The listing builds one solid part. Answer for the finished solid, in the listing's coordinates (mm). A direction names the side the tool comes from. Coordinates: 2 decimals unless noted, no trailing zeros. Order: outer loops, then holes, each group sorted by start corner. A loop starts at its lowest first (then second) coordinate and runs counter-clockwise, first axis right, second up. Notation, with made-up numbers: (-16, 42.5) -> (33, 42.5) arc R13 cw to (33, 66.5) -> close; hole circle Ø9 at (-14, -30). An arc over 180 degrees is marked (long way). Write item = value, one per line.
from build123d import *

# Parameters (mm, degrees)
CYLINDER127_R             = 1.6
CYLINDER127_DEPTH         = 25
CYLINDER126_R             = 1.6
CYLINDER126_DEPTH         = 25
CYLINDER128_R             = 1.6
CYLINDER128_DEPTH         = 25
CYLINDER129_R             = 1.6
CYLINDER129_DEPTH         = 25
FUSION106_PLACEMENT_ANGLE = 3
BOX058_W                  = 8
BOX058_H                  = 8
BOX058_DEPTH              = 50
BOX057_W                  = 110
BOX057_H                  = 10
BOX057_DEPTH              = 10
BOX059_W                  = 10
BOX059_H                  = 10
BOX059_DEPTH              = 50
BOX056_W                  = 110
BOX056_H                  = 10
BOX056_DEPTH              = 10
FILLET026_R               = 9.99
FILLET026_PLACEMENT_ANGLE = 3


with BuildPart() as cylinder127:
    # Cylinder127 → Cylinder127 (new body)
    with BuildSketch(Plane(origin=(76.5, 96, 46.5), x_dir=(1, 0, 0), z_dir=(0, -1, 0))):
        Circle(CYLINDER127_R)
    extrude(amount=CYLINDER127_DEPTH)


with BuildPart() as cylinder126:
    # Cylinder126 → Cylinder126 (new body)
    with BuildSketch(Plane(origin=(76.5, 96, 3.5), x_dir=(1, 0, 0), z_dir=(0, -1, 0))):
        Circle(CYLINDER126_R)
    extrude(amount=CYLINDER126_DEPTH)


with BuildPart() as cylinder128:
    # Cylinder128 → Cylinder128 (new body)
    with BuildSketch(Plane(origin=(3.5, 96, 46.5), x_dir=(1, 0, 0), z_dir=(0, -1, 0))):
        Circle(CYLINDER128_R)
    extrude(amount=CYLINDER128_DEPTH)


with BuildPart() as fusion106:
    # Cylinder129 → Cylinder129 (new body)
    with BuildSketch(Plane(origin=(3.5, 96, 3.5), x_dir=(1, 0, 0), z_dir=(0, -1, 0))):
        Circle(CYLINDER129_R)
    extrude(amount=CYLINDER129_DEPTH)

    # Fusion106: union Cylinder127, Cylinder126, Cylinder128
    add(cylinder127.part)
    add(cylinder126.part)
    add(cylinder128.part)


with BuildPart() as fusion106_1:
    # Fusion106 placement: moved
    add(fusion106.part.moved(Location((306, -120, -55))).rotate(Axis((306, -120, -55), (0, -1, 0)), FUSION106_PLACEMENT_ANGLE))


with BuildPart() as cube037:
    # Box058 → Box058 (new body)
    with BuildSketch(Plane(origin=(100, 2, -40), x_dir=(1, 0, 0), z_dir=(0, 0, 1))):
        with Locations((4, 4)):
            Rectangle(BOX058_W, BOX058_H)
    extrude(amount=BOX058_DEPTH)


with BuildPart() as cube036:
    # Box057 → Box057 (new body)
    with BuildSketch(Plane.XY.offset(-40)):
        with Locations((55, 5)):
            Rectangle(BOX057_W, BOX057_H)
    extrude(amount=BOX057_DEPTH)


with BuildPart() as cube038:
    # Box059 → Box059 (new body)
    with BuildSketch(Plane.XY.offset(-40)):
        with Locations((5, 5)):
            Rectangle(BOX059_W, BOX059_H)
    extrude(amount=BOX059_DEPTH)


with BuildPart() as cut067:
    # Box056 → Box056 (new body)
    with BuildSketch(Plane.XY):
        with Locations((55, 5)):
            Rectangle(BOX056_W, BOX056_H)
    extrude(amount=BOX056_DEPTH)

    # Fusion100: union Cube037, Cube036, Cube038
    add(cube037.part)
    add(cube036.part)
    add(cube038.part)

    # Fillet026
    fillet026_edges = [cut067.edges().sort_by_distance(p)[0] for p in [
        (0, 0, -15),
    ]]
    fillet(fillet026_edges, radius=FILLET026_R)


with BuildPart() as cut067_1:
    # Fillet026 placement: moved
    add(cut067.part.moved(Location((276, -49, -16))).rotate(Axis((276, -49, -16), (0, -1, 0)), FILLET026_PLACEMENT_ANGLE))

    # Cut067: cut Fusion106
    add(fusion106_1.part, mode=Mode.SUBTRACT)


with BuildPart() as cut067_2:
    # Cut067 placement: moved
    add(cut067_1.part.moved(Location((0, -5, 0))))


solid = cut067_2.part
Q1. A tool of negligible diameter and unlimited length cuts with its end or side. For faces 1 (the face through (376.66, -48.06, -25.96)), 2 (the face through (279.612, -50.996, -30.481)), from which of +Z, -Z, +X, -X, +Y, -Y can it reach the whole face along a straight path? Write none if from no direction.
The answers:
face_1 = +Y, -Y
face_2 = -Z, -X, -Y
Q2. Find the intervals of material crossed by line 1 along X through (y, z) = (-51.25, -38); line 2 along Z through (x, y) = (301.5, -51.75); line 3 along Z through (x, y) = (288.5, -53.25), in increasing order.
The answers:
line_1 = 280.26 to 287.17, 377.29 to 385.3
line_2 = -54.72 to -44.7, -14.66 to -4.65
line_3 = -55.4 to -45.39, -15.34 to -5.33
Q3. Section B-B, the plane y = -46.75 is taken. Give the vertices of the cut face in (x, z).
The answers:
outline = (275.86, -5.99) -> (278.48, -55.93) -> (387.94, -50.19) -> (387.42, -40.2) -> (385.42, -40.31) -> (383.85, -10.35) -> (385.85, -10.24) -> (385.33, -0.26) -> close; hole (285.99, -15.48) -> (287.56, -45.44) -> (377.43, -40.73) -> (375.86, -10.77) -> close; hole circle Ø3.2 at (307.06, -8.38); hole circle Ø3.2 at (309.31, -51.32); hole circle Ø3.2 at (379.96, -4.56); hole circle Ø3.2 at (382.21, -47.5)
Q4. Section A-A, the plane x = 303.5 is taken. Give the vertices of the cut face in (y, z).
The answers:
outline = (-54, -54.61) -> (-44, -54.61) -> (-44, -44.6) -> (-54, -44.6) -> close; (-54, -14.56) -> (-44, -14.56) -> (-44, -4.55) -> (-54, -4.55) -> close
Q5. The mould has two halves that part along Z. Classify faces 3 (the face through (332.249, -48.93, -53.107)), 4 (the face through (385.59, -49.07, -5.32)), 5 (the face through (380.612, -48.93, -47.514)): released by +Z, released by -Z, zero draft, split by the parting line, or undercut.
The answers:
face_3 = released by -Z
face_4 = released by +Z
face_5 = undercut
Q6. Each of these flat-tipped pins is pushed along its axis until it touches: pin 1 Ø6 at (x, y) = (346, -50.5) entering from -Z; pin 2 Ø2 at (x, y) = (319.5, -50) entering from +Z; pin 3 Ø10.5 at (x, z) = (381, -19) entering from -Y. Where does it stop, or does it pass through?
The answers:
pin_1 = -52.54
pin_2 = -3.65
pin_3 = -52
